Design review of the part built by this model. Coordinates are the model's own, in mm. Coordinates: 2 decimals unless noted, no trailing zeros. Write each loop counter-clockwise with the first axis right and the second up, starting at its lowest first coordinate (ties: lowest second). Pieces come first, ordered by that corner, then holes. Notation, with made-up numbers: M 60.5,46 L 112.5,46 A37 cw 112.5,84 Z; hole C -38,-30.75 d8. An arc over 180 degrees is marked long. Return JSON: item names as keys, results as strings. Group by question number.
```python
from build123d import *

# Parameters (mm, degrees)
SKETCH1_R           = 6.35
SKETCH1_R_2         = 3.5
BOSS_EXTRUDE1_DEPTH = 3.175


with BuildPart() as part:
    # Sketch1 → Boss-Extrude1 (new body)
    with BuildSketch(Plane.XY):
        with BuildLine():
            Line((-63.5, -25.4), (63.5, -25.4))
            Line((63.5, -25.4), (63.5, 177.8))
            ThreePointArc((63.5, 177.8), (48.491876086, 197.167012499), (25.991882686, 187.467772655))
            Line((25.991882686, 187.467772655), (-63.5, 25.4))
            Line((-63.5, 25.4), (-63.5, -25.4))
        make_face()
        with Locations((43.5, 177.8)):
            Circle(SKETCH1_R, mode=Mode.SUBTRACT)
        with Locations((-44.45, 12.7)):
            Circle(SKETCH1_R_2, mode=Mode.SUBTRACT)
        with Locations((44.45, 12.7)):
            Circle(SKETCH1_R_2, mode=Mode.SUBTRACT)
        with Locations((44.45, -12.7)):
            Circle(SKETCH1_R_2, mode=Mode.SUBTRACT)
        with Locations((-44.45, -12.7)):
            Circle(SKETCH1_R_2, mode=Mode.SUBTRACT)
        with Locations((12.7, 12.7)):
            Circle(SKETCH1_R_2, mode=Mode.SUBTRACT)
        with Locations((12.7, -12.7)):
            Circle(SKETCH1_R_2, mode=Mode.SUBTRACT)
        with Locations((43.5, 114.3)):
            Circle(SKETCH1_R_2, mode=Mode.SUBTRACT)
    extrude(amount=BOSS_EXTRUDE1_DEPTH)


solid = part.part
```
Item 1: Add section A-A (z = 0.85). Count the separate pieces of the cut face and the enclosed holes in it, plus the area to 3 significant figures.
Item 2: Add section B-B (y = -12.7). Write out the cut boundary in (x, z) (3 decimals), plus the area to 3 significant figures.
Item 3: For line 1 (Y direction, x = 14, z = 1.8); line 2 (Y direction, x = -44.45, z = 1.9); line 3 (Y direction, x = 44.45, z = 1.3), list the stretches that pass through material, from the lowest coordinate up.
Item 4: The part is to be moulded in two halves that separate along Y. For faces 1 (the cylindrical face through (14.58, 15.65, 1.57)), 2 (the cylindrical face through (48.85, 197.07, 1.57)), 3 (the cylindrical face through (-47.947, -12.546, 1.565)), 4 (the flat face through (13, 63, 3.175)), say which applies: pulls with the +Y half, pulls with the -Y half, needs draft (parallel to the pull), parting line crosses it, or undercut.
Item 5: Add section C-C (y = 114.3). Write out the cut boundary in (x, z) (3 decimals).
Item 6: For pin 1 (14.5 mm diameter, centred on x = 43.5, y = 177.8, fed in from -Z); pin 2 (6.5 mm diameter, centred on x = 12.7, y = -12.7, fed in from -Z), all flat-tipped, find the tip position at first contact; note any pin that passes through.
Item 7: Add section D-D (x = 12.7). Write out the cut boundary in (y, z) (3 decimals), plus the area to 3 significant figures.
Geometry check:
{
 "1": {"separate pieces": "1", "enclosed holes": "8", "area": "19,600 mm^2"},
 "2": {"outline": "M -63.5,0 L -47.95,0 L -47.95,3.175 L -63.5,3.175 Z; M -40.95,0 L 9.2,0 L 9.2,3.175 L -40.95,3.175 Z; M 16.2,0 L 40.95,0 L 40.95,3.175 L 16.2,3.175 Z; M 47.95,0 L 63.5,0 L 63.5,3.175 L 47.95,3.175 Z", "area": "337 mm^2"},
 "3": {"line 1": "-25.4 to -15.95, -9.45 to 9.45, 15.95 to 165.75", "line 2": "-25.4 to -16.2, -9.2 to 9.2, 16.2 to 59.9", "line 3": "-25.4 to -16.2, -9.2 to 9.2, 16.2 to 110.93, 117.67 to 171.52, 184.08 to 197.78"},
 "4": {"face 1": "undercut", "face 2": "pulls with the +Y half", "face 3": "undercut", "face 4": "needs draft"},
 "5": {"outline": "M -14.41,0 L 40,0 L 40,3.175 L -14.41,3.175 Z; M 47,0 L 63.5,0 L 63.5,3.175 L 47,3.175 Z"},
 "6": {"pin 1": "z = 0", "pin 2": "through"},
 "7": {"outline": "M -25.4,0 L -16.2,0 L -16.2,3.175 L -25.4,3.175 Z; M -9.2,0 L 9.2,0 L 9.2,3.175 L -9.2,3.175 Z; M 16.2,0 L 163.396,0 L 163.396,3.175 L 16.2,3.175 Z", "area": "555 mm^2"}
}
